Source: CAD feature listing. Evaluate the final solid. Frame: model axes, mm. Coordinates: 2 decimals unless noted, no trailing zeros. Order: outer loops, then holes, each group sorted by start corner. A loop starts at its lowest first (then second) coordinate and runs counter-clockwise, first axis right, second up. Notation, with made-up numbers: (-9, -19.75) -> (21, -19.75) arc R19 ccw to (21, -6.75) -> close; hole circle Ø5 at (20, 60.25). An arc over 180 degrees is marked (long way). Write item = value, one per line. Start each with the question number.
Item 1: Contact query for flat-ended pins moving along their axis: pin 1 (6 mm diameter, centred on y = -12, z = 33, fed in from -X); pin 2 (4 mm diameter, centred on x = 9, z = 10, fed in from -Y); pin 3 (10 mm diameter, centred on x = 835.5, z = 17.5, fed in from -Y); pin 4 (8 mm diameter, centred on y = -12.7, z = 50.8, fed in from -X). Output: stop coordinate, or through.
Item 2: Ray query, line 1 along X through (y, z) = (-3, 50.5); line 2 along Z through (x, y) = (22, -12.7); line 3 along Y through (x, z) = (31.5, 50.8). Return the intervals inside material, ascending. Write a range as [from, to].
Item 3: Section query B-B (z = 12). Output: boundary loops of the cut face in (x, y).
Item 4: Section query A-A (y = -12.7). Output: boundary loops of the cut face in (x, z) (3 decimals), then the cut area to 3 significant figures.
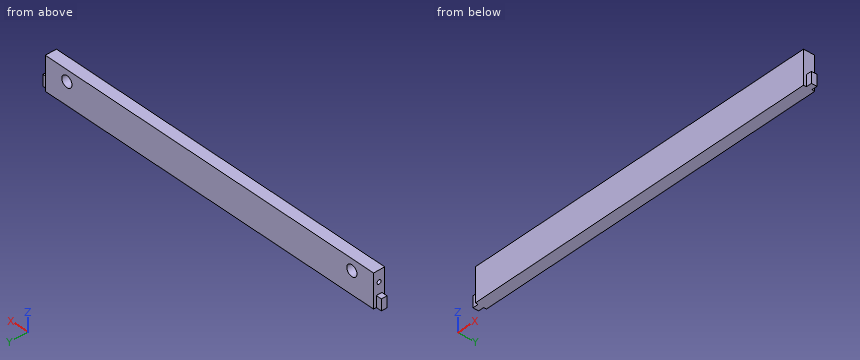
```python
from build123d import *

# Parameters (mm, degrees)
F0_W     = 844.55
F0_H     = 76.2
F1_DEPTH = 25.4
F2_W     = 12.7
F2_H     = 50.8
F3_DEPTH = 25.401
F4_W     = 12.7
F4_H     = 6.35
F5_DEPTH = 76.201
F6_R     = 4.564063
F7_DEPTH = 50.8
F8_R     = 12.7
F9_DEPTH = 19.05


with BuildPart() as f1:
    # F0 (on Front) → F1 (new body)
    with BuildSketch(Plane.XZ):
        with Locations((422.275, 38.1)):
            Rectangle(F0_W, F0_H)
    extrude(amount=F1_DEPTH)

    # F2 (on face) → F3 (cut, through all)
    with BuildSketch(Plane.XZ.offset(25.4)):
        with Locations((6.35, 50.8)):
            Rectangle(F2_W, F2_H)
        with Locations((838.2, 50.8)):
            Rectangle(F2_W, F2_H)
    extrude(amount=-F3_DEPTH, mode=Mode.SUBTRACT)

    # F4 (on face) → F5 (cut, through all)
    with BuildSketch(Plane(origin=(0, 0, 0), x_dir=(1, 0, 0), z_dir=(0, 0, -1))):
        with Locations((838.2, 22.225)):
            Rectangle(F4_W, F4_H)
        with Locations((838.2, 3.175)):
            Rectangle(F4_W, F4_H)
        with Locations((6.35, 22.225)):
            Rectangle(F4_W, F4_H)
        with Locations((6.35, 3.175)):
            Rectangle(F4_W, F4_H)
    extrude(amount=-F5_DEPTH, mode=Mode.SUBTRACT)

    # F6 (on face) → F7 (cut)
    with BuildSketch(Plane(origin=(12.7, 0, 0), x_dir=(0, -1, 0), z_dir=(-1, 0, 0))):
        with Locations((12.7, 50.8)):
            Circle(F6_R)
    extrude(amount=-F7_DEPTH, mode=Mode.SUBTRACT)

    # F8 (on face) → F9 (cut)
    with BuildSketch(Plane(origin=(0, 0, 0), x_dir=(-1, 0, 0), z_dir=(0, 1, 0))):
        with Locations((-66.675, 50.8)):
            Circle(F8_R)
        with Locations((-777.875, 50.8)):
            Circle(F8_R)
    extrude(amount=-F9_DEPTH, mode=Mode.SUBTRACT)


solid = f1.part
```
Computed:
q1.pin_1 = 12.7
q1.pin_2 = -19.05
q1.pin_3 = -25.4
q1.pin_4 = 78.73
q2.line_1 = [12.7, 53.98], [79.37, 765.18], [790.57, 831.85]
q2.line_2 = [0, 46.24], [55.36, 76.2]
q2.line_3 = [-25.4, -17.26], [-8.14, 0]
q3.outline = (0, -19.05) -> (12.7, -19.05) -> (12.7, -25.4) -> (831.85, -25.4) -> (831.85, -19.05) -> (844.55, -19.05) -> (844.55, -6.35) -> (831.85, -6.35) -> (831.85, 0) -> (12.7, 0) -> (12.7, -6.35) -> (0, -6.35) -> close
q4.outline = (0, 0) -> (844.55, 0) -> (844.55, 25.4) -> (831.85, 25.4) -> (831.85, 76.2) -> (12.7, 76.2) -> (12.7, 55.364) -> (54.823, 55.364) arc R12.7 cw (long way) to (54.823, 46.236) -> (12.7, 46.236) -> (12.7, 25.4) -> (0, 25.4) -> close; hole circle Ø25.4 at (777.875, 50.8)
q4.area = 61,700 mm^2
